from build123d import *

# Parameters (mm, degrees)
F1_DEPTH = 4
F2_R     = 1.6
F3_DEPTH = 4.001
F4_R     = 1
F5_DEPTH = 4.001


with BuildPart() as f1:
    # F0 (on Front) → F1 (new body)
    with BuildSketch(Plane.XZ):
        with BuildLine():
            Line((-4, 5.765), (-10.199683, 3.815857))
            ThreePointArc((-10.199683, 3.815857), (-13, 0), (-10.199683, -3.815857))
            Line((-10.199683, -3.815857), (-4, -5.765))
            Line((-4, -5.765), (4, -5.765))
            Line((4, -5.765), (10.199683, -3.815857))
            ThreePointArc((10.199683, -3.815857), (13, 0), (10.199683, 3.815857))
            Line((10.199683, 3.815857), (4, 5.765))
            Line((4, 5.765), (-4, 5.765))
        make_face()
    extrude(amount=F1_DEPTH)

    # F2 (on face) → F3 (cut, through all)
    with BuildSketch(Plane.XZ.offset(4)):
        with Locations((-9, 0)):
            Circle(F2_R)
        with Locations((9, 0)):
            Circle(F2_R)
    extrude(amount=-F3_DEPTH, mode=Mode.SUBTRACT)

    # F4 (on face) → F5 (cut, through all)
    with BuildSketch(Plane.XZ.offset(4)):
        Circle(F4_R)
    extrude(amount=-F5_DEPTH, mode=Mode.SUBTRACT)


solid = f1.part
The listing builds one solid part. Answer for the finished solid, in the listing's coordinates (mm). Coordinates: 2 decimals unless noted, no trailing zeros. Loops run counter-clockwise (first coordinate to the right, second up) from the corner with the lowest first, then second, coordinate; pieces in that order, holes last.
1) Determine the mould class of faces 1 (the face through (-7.143, -1.972, -4.777)), 2 (the face through (13, -2, 0)), 3 (the face through (7.4, -2.03, 0.07)), 4 (the face through (-0.2, 0, -1.2)) for opening direction X: pulls with the +X half, pulls with the -X half, needs draft (parallel to the pull), parting line crosses it, or undercut.
2) Find section B-B on x = 0. Write down the section's boundary in (y, z) (3 decimals), then the cut area to 3 significant figures.
3) Find section C-C on y = -1.2. Write down the section's boundary in (x, z) (3 decimals).
4) A flat-ended cylindrical pin translates along its axis: pin 1 Ø3.5 at (x, z) = (-9, 0) entering from +Y. Find the tip coordinate at first contact, or state that the pin passes through.
5) Find the intervals of material crossed by L1, parallel to X at y = -1.3, z = 1.25; L2, parallel to Z at x = 0, y = -1.65 (3 decimals); L3, parallel to Z at x = -9, y = -3, in increasing order.
6) Find section D-D on x = 8.75. Write down the section's boundary in (y, z), then the cut area to 3 significant figures.
7) Find section A-A on z = 0. Write down the section's boundary in (x, y).
Values:
1. face 1: pulls with the -X half
1. face 2: pulls with the +X half
1. face 3: undercut
1. face 4: needs draft
2. outline: (-4, -5.765) - (0, -5.765) - (0, -1) - (-4, -1) - close; (-4, 1) - (0, 1) - (0, 5.765) - (-4, 5.765) - close
2. area: 38.1 mm2
3. outline: (-10.2, -3.816) - (-4, -5.765) - (4, -5.765) - (10.2, -3.816) arc R4 ccw to (10.2, 3.816) - (4, 5.765) - (-4, 5.765) - (-10.2, 3.816) arc R4 ccw to start; hole circle Ø3.2 at (-9, 0); hole circle Ø2 at (0, 0); hole circle Ø3.2 at (9, 0)
4. pin 1: stops at y = 0
5. L1: x = -12.8 to -10, -8 to 8, 10 to 12.8
5. L2: z = -5.765 to -1, 1 to 5.765
5. L3: z = -4.19 to -1.6, 1.6 to 4.19
6. outline: (-4, -4.27) - (0, -4.27) - (0, -1.58) - (-4, -1.58) - close; (-4, 1.58) - (0, 1.58) - (0, 4.27) - (-4, 4.27) - close
6. area: 21.5 mm2
7. outline: (-13, -4) - (-10.6, -4) - (-10.6, 0) - (-13, 0) - close; (-7.4, -4) - (-1, -4) - (-1, 0) - (-7.4, 0) - close; (1, -4) - (7.4, -4) - (7.4, 0) - (1, 0) - close; (10.6, -4) - (13, -4) - (13, 0) - (10.6, 0) - close
